Source: CAD feature listing. Evaluate the final solid. Frame: model axes, mm. Face numbers are marked on the shaded views. A direction names the side the tool comes from. Give positions to 0.01 mm unless a question says otherwise; leave off trailing zeros. Order: outer loops, then holes, each group sorted by start corner. A loop starts at its lowest first (then second) coordinate and runs counter-clockwise, first axis right, second up. Notation, with made-up numbers: (67.5, 40.25) - (125.5, 40.25) arc R12 ccw to (125.5, 63.25) - close; hole circle Ø9 at (-13, 60.25). An arc over 180 degrees is marked (long way). Use CSV: the item, a comma, the result in double quotes.
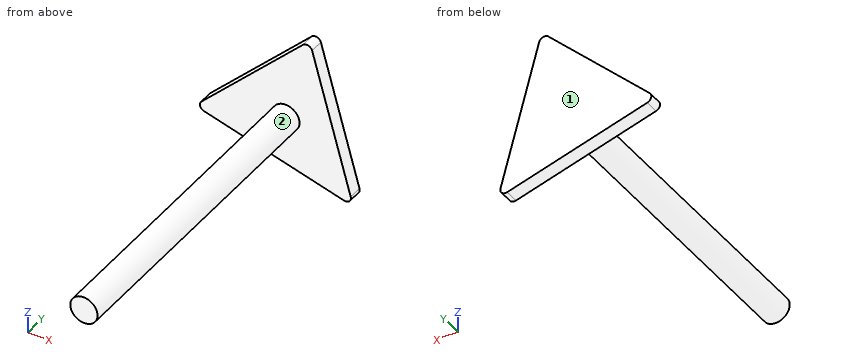
```python
from build123d import *

# Parameters (mm, degrees)
F0_R     = 12.7
F1_DEPTH = 304.8
F2_DEPTH = 12.7
F3_R     = 5.08


with BuildPart() as f1:
    # F0 (on Front) → F1 (new body)
    with BuildSketch(Plane.XZ):
        Circle(F0_R)
    extrude(amount=F1_DEPTH)

    # F0 (on Front) → F2 (join)
    with BuildSketch(Plane.XZ):
        Polygon((62.721773, -61.708178), (22.079963, 85.172738), (-84.801736, -23.46456), align=None)
        Circle(F0_R, mode=Mode.SUBTRACT)
    extrude(amount=F2_DEPTH)

    # F3
    f3_edges = [f1.edges().sort_by_distance(p)[0] for p in [
        (-84.801736, -6.35, -23.46456),
        (22.079963, -6.35, 85.172738),
        (62.721773, -6.35, -61.708178),
    ]]
    fillet(f3_edges, radius=F3_R)


solid = f1.part
```
Item 1: Section B-B on x = 0. Return the cut outline in (y, z), then the cut area to 3 significant figures.
Filled in:
outline,"(-304.8, -12.7) - (-12.7, -12.7) - (-12.7, -45.45) - (0, -45.45) - (0, 62.73) - (-12.7, 62.73) - (-12.7, 12.7) - (-304.8, 12.7) - close"
area,"8,790 mm2"
Item 2: Set-up query: the marked faces 1 and 2. Return all of +Z, -Z, +X, -X, +Y, -Y with unobstructed straight access to the full face (end or side cutting, diameter ignored); none if empty.
Filled in:
face 1,"+Z, -Z, +X, -X, +Y"
face 2,"-Y"
Item 3: First-contact query: pin 1 (2 mm diameter, centred on x = 20.5, z = -4, fed in from -Y); pin 2 (6 mm diameter, centred on x = 3.5, y = -176, fed in from +Z); pin 3 (6 mm diameter, centred on y = -116, z = -13.5, fed in from +X). Flat tips, straight axial feed; report the tip coordinate or a pass-through.
Filled in:
pin 1,"stops at y = -12.7"
pin 2,"stops at z = 12.69"
pin 3,"stops at x = 7.14"
Item 4: Section D-D on x = -50. Return the cut outline in (y, z), then the cut area to 3 significant figures.
Filled in:
outline,"(-12.7, -32.49) - (0, -32.49) - (0, 11.91) - (-12.7, 11.91) - close"
area,"564 mm2"
Item 5: Section C-C on z = -8. Return the cut outline in (x, y), then the cut area to 3 significant figures.
Filled in:
outline,"(-69.59, -12.7) - (-9.86, -12.7) - (-9.86, -304.8) - (9.86, -304.8) - (9.86, -12.7) - (47.86, -12.7) - (47.86, 0) - (-69.59, 0) - close"
area,"7,250 mm2"
Item 6: Section A-A on y = -126.5. Return the cut outline in (x, z), then the cut area to 3 significant figures.
Filled in:
outline,"circle Ø25.4 at (0, 0)"
area,"507 mm2"
Item 7: Material intervals for line 1 (Y direction, x = 22.5, z = 74.5); line 2 (Z direction, x = 11, y = -111); line 3 (X direction, y = -167.5, z = 4), sorted ascending. Write a range as from..to.
Filled in:
line 1,"y = -12.7..0"
line 2,"z = -6.35..6.35"
line 3,"x = -12.05..12.05"
